from build123d import *
from build123d.topology import SkipClean

# Parameters (mm, degrees)
SKETCH2_R           = 4
BOSS_EXTRUDE1_DEPTH = 66.9
BOSS_EXTRUDE2_DEPTH = 7.5
SKETCH4_W           = 1
SKETCH4_H           = 0.5


with BuildPart() as part:
    # Sketch2 → Boss-Extrude1 (new body)
    with BuildSketch(Plane(origin=(0, 0, 0), x_dir=(0, 0, -1), z_dir=(1, 0, 0))):
        with Locations(Location((0, 0, 0), (0, 0, 180))):
            Circle(SKETCH2_R)
    extrude(amount=BOSS_EXTRUDE1_DEPTH)

    # Sketch3 → Boss-Extrude2 (add)
    with SkipClean():  # the faces are left unmerged after this step: merging them gives an invalid solid
        with BuildSketch(Plane(origin=(66.9, 0, 0), x_dir=(0, 0, -1), z_dir=(1, 0, 0))):
            with BuildLine():
                Line((-3.469855905, 1.99), (3.469855905, 1.99))
                ThreePointArc((3.469855905, 1.99), (0, -4), (-3.469855905, 1.99))
            make_face()
        extrude(amount=BOSS_EXTRUDE2_DEPTH)

    # Sketch4 → Cut-Revolve1 (revolve, cut)
    with SkipClean():  # the faces are left unmerged after this step: merging them gives an invalid solid
        with BuildSketch(Plane.XY, mode=Mode.PRIVATE) as cut_revolve1_sk:
            with Locations((1.5, 3.75)):
                Rectangle(SKETCH4_W, SKETCH4_H)
        revolve(cut_revolve1_sk.sketch.rotate(Axis((0, 0, 0), (1, 0, 0)), 90), axis=Axis((0, 0, 0), (1, 0, 0)), mode=Mode.SUBTRACT)


solid = part.part
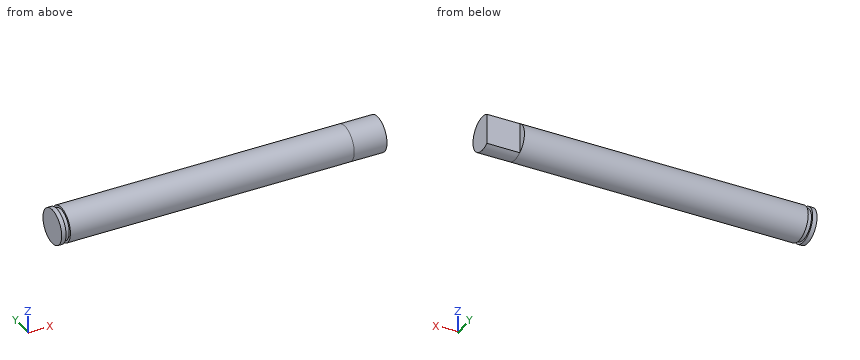
The model under review builds one solid part; all positions refer to its coordinate system, in mm. Coordinates: 2 decimals unless noted, no trailing zeros. Loops run counter-clockwise (first coordinate to the right, second up) from the corner with the lowest first, then second, coordinate; pieces in that order, holes last.
(1) Consider section C-C, the plane x = 68. Give the boundary of the cut face in (y, z).
Determined:
outline: (1.99, -3.47) - (1.99, 3.47) arc R4 ccw (long way) to start
(2) Consider section A-A, the plane z = 0. Give the boundary of the cut face in (x, y), plus the area to 3 significant figures.
Determined:
outline: (0, -4) - (1, -4) - (1, -3.5) - (2, -3.5) - (2, -4) - (74.4, -4) - (74.4, 1.99) - (66.9, 1.99) - (66.9, 4) - (2, 4) - (2, 3.5) - (1, 3.5) - (1, 4) - (0, 4) - close
area: 579 mm2
(3) Insertion check: P1, Ø2, axis at x = 34, z = -1.5, coming from the -Y side; P2, Ø3, axis at x = 64.5, z = 2, coming from the +Y side; P3, Ø2, axis at x = 43, z = -3, coming from the -Y side. Each pin has a flat end and moves straight along its axis. Give the tip position at first contact, or say it passes through.
Determined:
P1: stops at y = -3.97
P2: stops at y = 3.97
P3: stops at y = -3.46
(4) Wall thickness on L1, parallel to X at y = -3.5, z = 0.5; L2, parallel to X at y = 2.5, z = -2.5; L3, parallel to Z at x = 67, y = -0.25: over which ranges is each line inside the solid? List them lowest first.
Determined:
L1: x = 0 to 1, 2 to 74.4
L2: x = 0 to 1, 2 to 66.9
L3: z = -3.99 to 3.99
(5) Consider section D-D, the plane x = 36. Give the boundary of the cut face in (y, z), plus the area to 3 significant figures.
Determined:
outline: circle Ø8 at (0, 0)
area: 50.3 mm2
(6) Consider section B-B, the plane y = 0.75. Give the boundary of the cut face in (x, z), plus the area to 3 significant figures.
Determined:
outline: (0, -3.93) - (1, -3.93) - (1, -3.42) - (2, -3.42) - (2, -3.93) - (74.4, -3.93) - (74.4, 3.93) - (2, 3.93) - (2, 3.42) - (1, 3.42) - (1, 3.93) - (0, 3.93) - close
area: 584 mm2
